Autodesk Inventor part; units mm, degrees
ref_plane "YZ Plane" through (0, 0, 0) normal (1, 0, 0) x (0, 1, 0)
ref_plane "XZ Plane" through (0, 0, 0) normal (0, 1, 0) x (-1, 0, 0)
ref_plane "XY Plane" through (0, 0, 0) normal (0, 0, 1) x (1, 0, 0)
sketch "草圖1" plane through (0, 0, 0) normal (0, 1, 0) x (-1, 0, 0)
  line L0 (-50, 50) -> (50, 50)
  line L1 (50, 50) -> (50, -50)
  line L2 (50, -50) -> (-50, -50)
  line L3 (-50, -50) -> (-50, 50)
  line L4 (-50, 50) -> (50, -50) construction
  line L5 (50, 50) -> (-50, -50) construction
  point P0 (0, 0)
  dimension "d0" = 100
  dimension "d1" = 100
extrude "擠出1" add sketch "草圖1" against normal blind 50
shell "薄殼1" thickness 3 removed faces 1 at (-16.6667, -16.6667, 50)
sketch "草圖2" plane through (0, 0, 0) normal (0, 1, 0) x (1, 0, 0)
  line L0 (50, 50) -> (-50, 50) construction
  line L1 (-50, 50) -> (-50, -50) construction
  line L2 (-50, -50) -> (50, -50) construction
  line L3 (50, -50) -> (50, 50) construction
  line L4 (50, 50) -> (0, 50) construction
  line L5 (20, 30) -> (20, 0) construction
  line L6 (20, 0) -> (50, 0) construction
  line L7 (50, 0) -> (50, 50) construction
  circle A0 centre (20, 0) radius 30 construction
  line L8 (5.5, -6.25) -> (34.5, -6.25) construction
  line L9 (34.5, -6.25) -> (34.5, 6.25) construction
  line L10 (34.5, 6.25) -> (5.5, 6.25) construction
  line L11 (5.5, 6.25) -> (5.5, -6.25) construction
  line L12 (5.5, -6.25) -> (34.5, 6.25) construction
  line L13 (34.5, -6.25) -> (5.5, 6.25) construction
  circle A1 centre (5.5, 0) radius 1.25
  circle A2 centre (34.5, 0) radius 1.25
  point P0 (0, 0)
  dimension "d16" = 60
  dimension "d5" = 29
  dimension "d6" = 12.5
  dimension "d7" = 2.5
extrude "擠出2" cut sketch "草圖2" against normal up to surface (3 mm away)
sketch "草圖3" plane through (0, 0, 0) normal (0, 1, 0) x (1, 0, 0)
  line L0 (8, -6.25) -> (32, -6.25)
  line L1 (32, -6.25) -> (32, 6.25)
  line L2 (32, 6.25) -> (8, 6.25)
  line L3 (8, 6.25) -> (8, -6.25)
  line L4 (8, -6.25) -> (32, 6.25) construction
  line L5 (32, -6.25) -> (8, 6.25) construction
  line L6 (30.5, -3) -> (33.5, -3)
  line L7 (33.5, -3) -> (33.5, 3)
  line L8 (33.5, 3) -> (30.5, 3)
  line L9 (30.5, 3) -> (30.5, -3)
  line L10 (30.5, -3) -> (33.5, 3) construction
  line L11 (33.5, -3) -> (30.5, 3) construction
  point P0 (0, 0)
  point P1 (20, 0)
  point P2 (32, 0)
  point P3 (32, -3)
  point P4 (32, 3)
  dimension "d10" = 24
  dimension "d11" = 12.5
  dimension "d12" = 3
  dimension "d13" = 6
extrude "擠出3" cut sketch "草圖3" against normal up to surface (3 mm away)
properties part number "base_box"
Can you work these out from the model? Positions are in its coordinate system, mm. A direction names the side the tool comes from. Coordinates: 2 decimals unless noted, no trailing zeros. Order: outer loops, then holes, each group sorted by start corner. A loop starts at its lowest first (then second) coordinate and runs counter-clockwise, first axis right, second up. Notation, with made-up numbers: M -14,-0.5 L 33,-0.5 A26 cw 33,38.5 Z; hole C 62,38 d1. An arc over 180 degrees is marked long. Write item = value, one per line.
(1) For pin 1 Ø2 at (x, z) = (7.5, 5.5) entering from +Y, with a flat end and sliding along its axis, tell me the tip position at first contact or that it passes through.
Results are:
pin_1 = 0
(2) Suppose I cut it at A-A on x = 5.5. Please give me the cut outline in (y, z), plus the area to 4 significant figures.
Results are:
outline = M -50,-50 L 0,-50 L 0,-1.25 L -3,-1.25 L -3,-47 L -47,-47 L -47,50 L -50,50 Z; M -3,1.25 L 0,1.25 L 0,50 L -3,50 Z
area = 724.5 mm2
(3) Suppose I cut it at C-C on x = 41. Please give me the cut outline in (y, z), plus the area to 3 significant figures.
Results are:
outline = M -50,-50 L 0,-50 L 0,50 L -3,50 L -3,-47 L -47,-47 L -47,50 L -50,50 Z
area = 732 mm2
(4) Suppose I cut it at B-B on z = -13. Please give me the cut outline in (x, y), plus the area to 3 significant figures.
Results are:
outline = M -50,-50 L 50,-50 L 50,0 L -50,0 Z; hole M -47,-47 L 47,-47 L 47,-3 L -47,-3 Z
area = 864 mm2
(5) If we mould it in two halves opening along X, with no side actions, what happens to faces 1 (the face through (0, -49, 50)), 2 (the face through (50, -25, -1)), 3 (the face through (20, -1, 6.25))? For each: pulls with the +X half, pulls with the -X half, needs draft (parallel to the pull), parting line crosses it, or undercut.
Results are:
face_1 = needs draft
face_2 = pulls with the +X half
face_3 = undercut
(6) For faces 4 (the face through (1, -3, 2)), 5 (the face through (-50, -25, 1)), 6 (the face through (8, -1, 0)), which set-ups out of +Z, -Z, +X, -X, +Y, -Y let a thin tool reach every point of the face, with its end or its side?
Results are:
face_4 = +Z
face_5 = +Z, -Z, -X, +Y, -Y
face_6 = +Y
(7) I need wall thicknesses on line 1 along X through (y, z) = (-2, 0); line 2 along X through (y, z) = (-25, 8.5); line 3 along Y through (x, z) = (-10.5, 22). Which ranges of each line are inside material? Lowest first, please. Write a range as [from, to].
Results are:
line_1 = [-50, 4.25], [6.75, 8], [35.75, 50]
line_2 = [-50, -47], [47, 50]
line_3 = [-50, -47], [-3, 0]
(8) Suppose I cut it at D-D on y = -29. Please give me the cut outline in (x, z).
Results are:
outline = M -50,-50 L 50,-50 L 50,50 L 47,50 L 47,-47 L -47,-47 L -47,50 L -50,50 Z
